Answer from the drawing. Dimensions are ordinates in mm from the lowest x, y and z of the part. Coordinates: 2 decimals unless noted, no trailing zeros. Order: outer loops, then holes, each group sorted by start corner. A loop starts at its lowest first (then second) coordinate and runs counter-clockwise, first axis right, second up. Notation, with made-up numbers: (-17, 37.5) - (-9, 37.5) arc R20 cw to (-9, 76.5) - close; hole circle Ø5 at (21, 24). An arc over 180 degrees is marked (long way). Answer as a JSON object with one key per item and string values. Group by question number.
1) Each of these flat-tipped pins is pushed along its axis until it touches: P1, Ø4.5, axis at x = 11.5, y = 11.5, coming from the -Z side; P2, Ø6, axis at x = 13, z = 18, coming from the -Y side; P3, Ø5.5, axis at x = 7.85, y = 7.85, coming from the +Z side; P4, Ø1.5, axis at y = 6.5, z = 15, coming from the -X side. Where does it stop, or does it pass through?
2) Section A-A (y = 7.85) is taken. Give the vertices of the cut face in (x, z), plus the area to 3 significant figures.
3) The mould has two halves that part along Y. Classify the marked faces 1, 2 and 3: released by +Y, released by -Y, zero draft, split by the parting line, or undercut.
4) Section D-D (y = 14.25) is taken. Count the separate pieces of the cut face and the enclosed holes in it, plus the area to 3 significant figures.
5) Section C-C (z = 23.75) is taken. Give the vertices of the cut face in (x, y).
6) Find the intervals of material crossed by line 1 along Z through (x, y) = (6, 1.5); line 2 along Y through (x, z) = (7.85, 5.25), in increasing order.
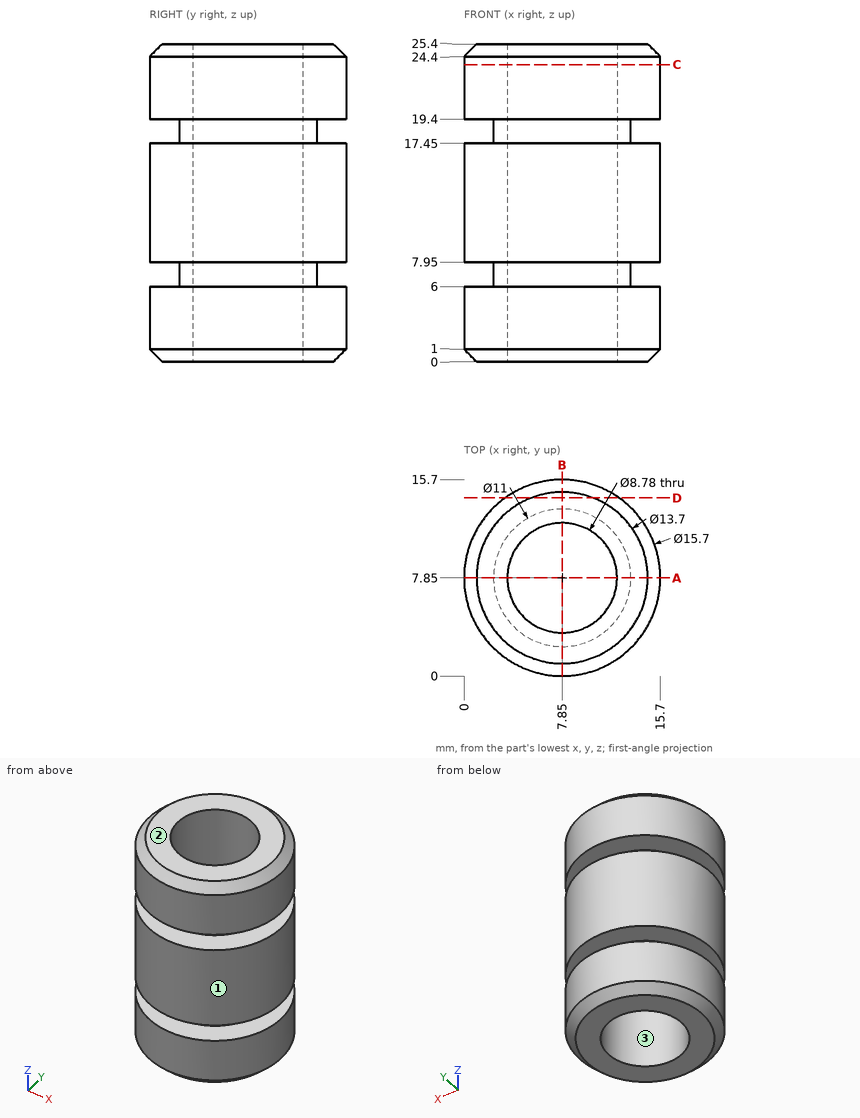
Report:
{
 "1": {"P1": "stops at z = 0", "P2": "stops at y = 0.31", "P3": "passes through", "P4": "stops at x = 0.02"},
 "2": {"outline": "(0, 1) - (1, 0) - (3.46, 0) - (3.46, 25.4) - (1, 25.4) - (0, 24.4) - (0, 19.4) - (2.35, 19.4) - (2.35, 17.45) - (0, 17.45) - (0, 7.95) - (2.35, 7.95) - (2.35, 6) - (0, 6) - close; (12.24, 0) - (14.7, 0) - (15.7, 1) - (15.7, 6) - (13.35, 6) - (13.35, 7.95) - (15.7, 7.95) - (15.7, 17.45) - (13.35, 17.45) - (13.35, 19.4) - (15.7, 19.4) - (15.7, 24.4) - (14.7, 25.4) - (12.24, 25.4) - close", "area": "155 mm²"},
 "3": {"face 1": "split by the parting line", "face 2": "zero draft", "face 3": "undercut"},
 "4": {"separate pieces": "3", "enclosed holes": "0", "area": "192 mm²"},
 "5": {"outline": "circle Ø15.7 at (7.85, 7.85); hole circle Ø8.78 at (7.85, 7.85)"},
 "6": {"line 1": "z = 0 to 6, 7.95 to 17.45, 19.4 to 25.4", "line 2": "y = 0 to 3.46, 12.24 to 15.7"}
}
